```python
from build123d import *

# Parameters (mm, degrees)
BOX3570_W        = 750
BOX3570_H        = 550
BOX3570_DEPTH    = 2150
BOX3572_W        = 500
BOX3572_H        = 550
BOX3572_DEPTH    = 500
ARRAY290_Z_COUNT = 4
ARRAY290_Z_PITCH = 550
BOX3571_W        = 1400
BOX3571_H        = 600
BOX3571_DEPTH    = 2200


with BuildPart() as box3570:
    # Box3570 → Box3570 (new body)
    with BuildSketch(Plane(origin=(8100, -300, 0), x_dir=(1, 0, 0), z_dir=(0, 0, 1))):
        with Locations((375, 275)):
            Rectangle(BOX3570_W, BOX3570_H)
    extrude(amount=BOX3570_DEPTH)


with BuildPart() as array290:
    # Box3572 → Box3572 (new body)
    with BuildSketch(Plane(origin=(7550, -300, 0), x_dir=(1, 0, 0), z_dir=(0, 0, 1))):
        with Locations((250, 275)):
            Rectangle(BOX3572_W, BOX3572_H)
    extrude(amount=BOX3572_DEPTH)

    # Array290 Z: Array290 ×4


with BuildPart() as array290_1:
    add(array290.part)
    with Locations(*[(0, 0, i * ARRAY290_Z_PITCH) for i in range(1, ARRAY290_Z_COUNT)]):
        add(array290.part)


with BuildPart() as cut006:
    # Box3571 → Box3571 (new body)
    with BuildSketch(Plane(origin=(7500, -300, 0), x_dir=(1, 0, 0), z_dir=(0, 0, 1))):
        with Locations((700, 300)):
            Rectangle(BOX3571_W, BOX3571_H)
    extrude(amount=BOX3571_DEPTH)

    # Cut007: cut Array290
    add(array290_1.part, mode=Mode.SUBTRACT)

    # Cut006: cut Box3570
    add(box3570.part, mode=Mode.SUBTRACT)


with BuildPart() as cut006_1:
    # Cut006 placement: moved
    add(cut006.part.moved(Location((-100, 0, 0))))


solid = cut006_1.part
```
Can you work these out from the model? Positions are in its coordinate system, mm. A direction names the side the tool comes from. Round coordinates to 2 decimals unless told otherwise and drop trailing zeros. Order: outer loops, then holes, each group sorted by start corner. A loop starts at its lowest first (then second) coordinate and runs counter-clockwise, first axis right, second up.
(1) On a 3-axis mill with a long thin cutter (end or side, diameter ignored), from which of +Z, -Z, +X, -X, +Y, -Y can I reach the whole of each face in a straight line? I mean faces 4 (the face through (7696, 250, 796)), 5 (the face through (8090, 4, 2200)), 6 (the face through (7950, -29, 246)). Say none if no direction works.
Results are:
face 4: -Y
face 5: +Z, +X, -X, +Y, -Y
face 6: -Z, -Y
(2) We'd pull the mould along X, two halves only. Please class faces 1 (the face through (7450, -29, 246)), 2 (the face through (7950, -29, 796)), 3 (the face through (8090, 300, 1085)): +X half, -X half, draft (parallel to the pull), parting line (faces both ways), or undercut.
Results are:
face 1: undercut
face 2: undercut
face 3: draft
(3) If we section it at A-A (y = -79): Please give me the cut outline in (x, z), plus the area to 4 significant figures.
Results are:
outline: (7400, 0) - (7450, 0) - (7450, 500) - (7950, 500) - (7950, 0) - (8000, 0) - (8000, 2150) - (8750, 2150) - (8750, 0) - (8800, 0) - (8800, 2200) - (7400, 2200) - close; hole (7450, 550) - (7950, 550) - (7950, 1050) - (7450, 1050) - close; hole (7450, 1100) - (7950, 1100) - (7950, 1600) - (7450, 1600) - close; hole (7450, 1650) - (7950, 1650) - (7950, 2150) - (7450, 2150) - close
area: 467,500 mm2
(4) If we section it at C-C (x = 8307.5): Please give me the cut outline in (y, z), plus the area to 4 significant figures.
Results are:
outline: (-300, 2150) - (250, 2150) - (250, 0) - (300, 0) - (300, 2200) - (-300, 2200) - close
area: 137,500 mm2
(5) If I drill on L1, parallel to X at y = 90.5, z = 1956.5; L2, parallel to Z at x = 7621.5, y = -200; L3, parallel to Y at x = 8491, z = 1493, over which ranges is the centre line in solid material (lowest first)?
Results are:
L1: x = 7400 to 7450, 7950 to 8000, 8750 to 8800
L2: z = 500 to 550, 1050 to 1100, 1600 to 1650, 2150 to 2200
L3: y = 250 to 300
(6) I'm going to push a flat-ended pin straight in: pin 1 (3 mm diameter, centred on x = 8122.5, y = 43, fed in from -Z). Where does the tip first touch, or does it pass through?
Results are:
pin 1: stops at z = 2150
(7) If we section it at B-B (z = 1536.5): Please give me the cut outline in (x, y), plus the area to 4 significant figures.
Results are:
outline: (7400, -300) - (7450, -300) - (7450, 250) - (7950, 250) - (7950, -300) - (8000, -300) - (8000, 250) - (8750, 250) - (8750, -300) - (8800, -300) - (8800, 300) - (7400, 300) - close
area: 152,500 mm2
